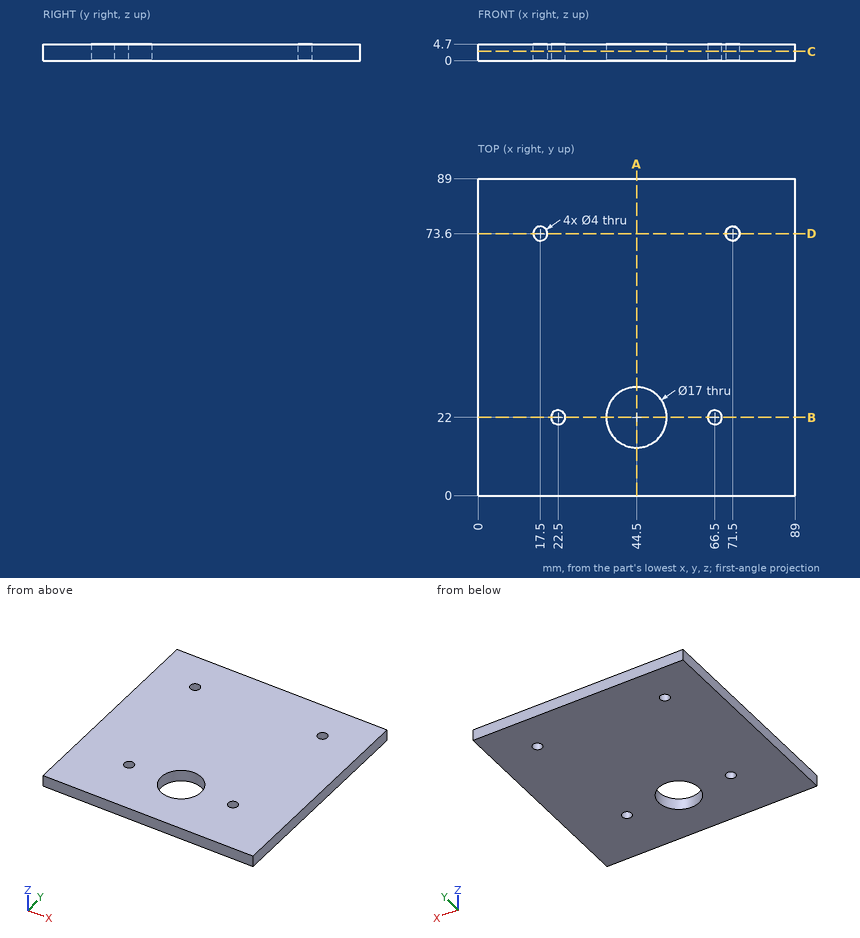
Can you work these out from the drawing? Everything is in mm from the part's minimum corner. Give positions to 0.01 mm unless a question says otherwise; leave off trailing zeros. Loops run counter-clockwise (first coordinate to the right, second up) from the corner with the lowest first, then second, coordinate; pieces in that order, holes last. Notation, with made-up numbers: (-28.5, 32.5) -> (27.5, 32.5) arc R21 ccw to (27.5, 53.5) -> close; hole circle Ø3 at (-12.75, 13). An arc over 180 degrees is marked (long way). Put each result on its own line as item: value.
(1) I'm going to push a flat-ended pin straight in: pin 1 Ø3.5 at (x, y) = (22.5, 22) entering from +Z. Where does the tip first touch, or does it pass through?
Computed:
pin 1: through
(2) Imagine slicing it at A-A on x = 44.5. Write out the boundary of the cut face in (y, z).
Computed:
outline: (0, 0) -> (13.5, 0) -> (13.5, 4.7) -> (0, 4.7) -> close; (30.5, 0) -> (89, 0) -> (89, 4.7) -> (30.5, 4.7) -> close
(3) Imagine slicing it at C-C on z = 2.65. Write out the boundary of the cut face in (x, y), plus the area to 3 significant figures.
Computed:
outline: (0, 0) -> (89, 0) -> (89, 89) -> (0, 89) -> close; hole circle Ø4 at (17.5, 73.6); hole circle Ø4 at (22.5, 22); hole circle Ø17 at (44.5, 22); hole circle Ø4 at (66.5, 22); hole circle Ø4 at (71.5, 73.6)
area: 7,640 mm^2
(4) Imagine slicing it at B-B on y = 22. Write out the boundary of the cut face in (x, z), plus the area to 3 significant figures.
Computed:
outline: (0, 0) -> (20.5, 0) -> (20.5, 4.7) -> (0, 4.7) -> close; (24.5, 0) -> (36, 0) -> (36, 4.7) -> (24.5, 4.7) -> close; (53, 0) -> (64.5, 0) -> (64.5, 4.7) -> (53, 4.7) -> close; (68.5, 0) -> (89, 0) -> (89, 4.7) -> (68.5, 4.7) -> close
area: 301 mm^2
(5) Imagine slicing it at D-D on y = 73.6. Write out the boundary of the cut face in (x, z).
Computed:
outline: (0, 0) -> (15.5, 0) -> (15.5, 4.7) -> (0, 4.7) -> close; (19.5, 0) -> (69.5, 0) -> (69.5, 4.7) -> (19.5, 4.7) -> close; (73.5, 0) -> (89, 0) -> (89, 4.7) -> (73.5, 4.7) -> close
(6) Please list where these lines run through material, in increasing order: probe 1 along Y at (x, z) = (17.5, 2.2); probe 2 along Y at (x, z) = (66.5, 3.2); probe 3 along X at (y, z) = (29, 2.7). Write a range as [from, to].
Computed:
probe 1: [0, 71.6], [75.6, 89]
probe 2: [0, 20], [24, 89]
probe 3: [0, 39.68], [49.32, 89]
